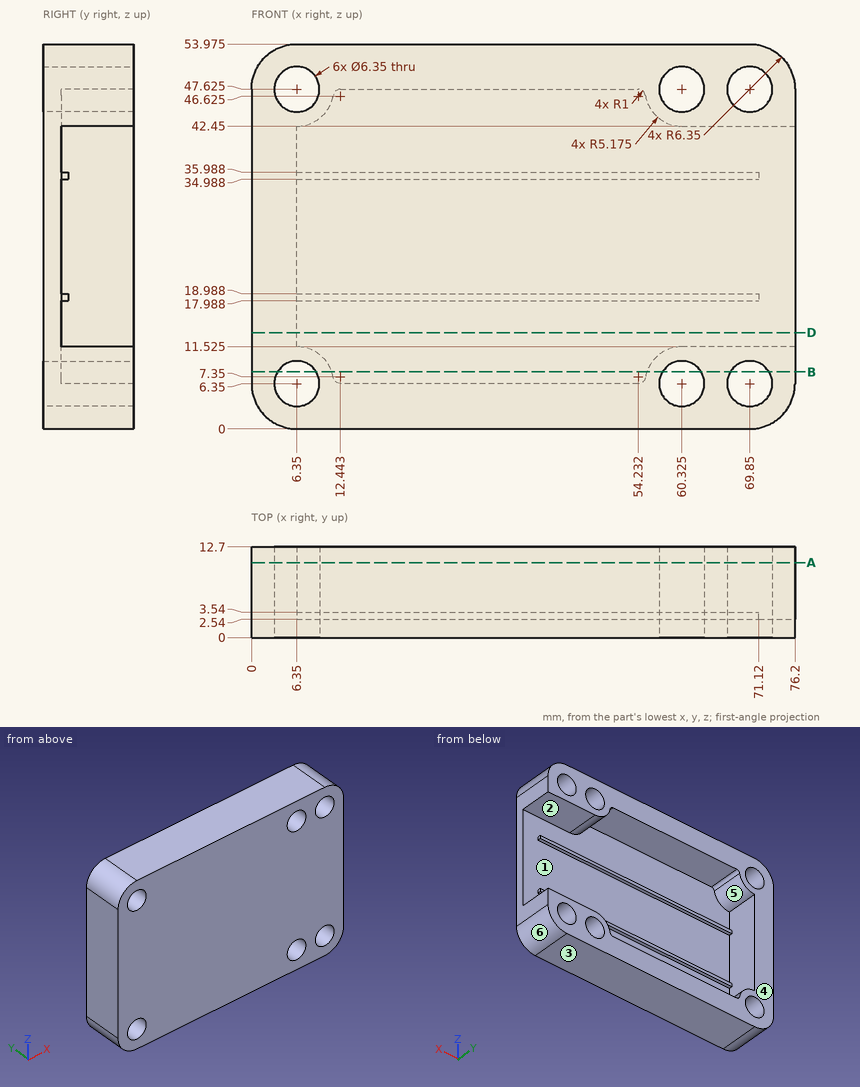
For this review, use the dimensioned drawing (mm, ordinates from the lowest corner) and the shaded views. A direction names the side the tool comes from. Give positions to 0.01 mm unless a question says otherwise; leave off trailing zeros. Loops run counter-clockwise (first coordinate to the right, second up) from the corner with the lowest first, then second, coordinate; pieces in that order, holes last. Notation, with made-up numbers: (58.25, 11) -> (94.25, 11) arc R16 cw to (94.25, 17) -> close; hole circle Ø2 at (31, -18.75). An arc over 180 degrees is marked (long way). One line per question, with ' | ' between items. Start each with the question number.
(1) We need section B-B (z = 8). State the section outline as (x, y) points (1 decimal).
(2) Draft analysis for pull direction X (two halves, no side actions). For the marked faces 4, 5 and 6, state which applies: +X half, -X half, draft (parallel to the pull), parting line (faces both ways), or undercut.
(3) We need section D-D (z = 13.5). State the section outline as (x, y) points.
(4) For line 1 (X direction, y = 9.75, z = 9) (1 decimal); line 2 (X direction, y = 11.25, z = 48); line 3 (X direction, y = 8.5, z = 30), list the stretches that pass through material, from the lowest coordinate up.
(5) We need section A-A (y = 10.5). State how many separate pieces and enclosed holes the cut face has, and give its area (3 significant figures).
(6) Insertion check: P1, Ø4, axis at x = 6.35, z = 47.625, coming from the -Y side; P2, Ø0.5, axis at y = 3, z = 18.5, coming from the +X side; P3, Ø6, axis at x = 17.5, z = 12.5, coming from the +Y side; P4, Ø0.8, axis at x = 32, z = 18.5, coming from the +Y side. Each pin has a flat end and moves straight along its axis. Give the tip position at first contact, or say it passes through.
(7) For the marked faces 1, 2 and 3, list the 3-axis set-ups (+Z, -Z, +X, -X, +Y, -Y) from which the entire face can be reached by the end or side of a thin tool; tool diameter is ignored.
The answers:
1) outline: (0, 0) -> (3.6, 0) -> (3.6, 12.7) -> (0, 12.7) -> close; (9.1, 0) -> (57.6, 0) -> (57.6, 12.7) -> (55.4, 12.7) -> (55.4, 2.5) -> (11.3, 2.5) -> (11.3, 12.7) -> (9.1, 12.7) -> close; (63, 0) -> (67.1, 0) -> (67.1, 12.7) -> (63, 12.7) -> close; (72.6, 0) -> (76.2, 0) -> (76.2, 12.7) -> (72.6, 12.7) -> close
2) face 4: draft | face 5: undercut | face 6: +X half
3) outline: (0, 0) -> (76.2, 0) -> (76.2, 2.54) -> (6.35, 2.54) -> (6.35, 12.7) -> (0, 12.7) -> close
4) line 1: x = 0 to 4.6, 8.1 to 10.8, 55.9 to 58.6, 62.1 to 68.1, 71.6 to 76.2 | line 2: x = 0.01 to 3.2, 9.5 to 57.17, 63.48 to 66.7, 73 to 76.19 | line 3: x = 0 to 6.35
5) separate pieces: 1 | enclosed holes: 6 | area: 1,250 mm^2
6) P1: passes through | P2: stops at x = 71.12 | P3: stops at y = 2.54 | P4: stops at y = 3.54
7) face 1: +Y | face 2: +X, +Y | face 3: -Z, +X, -X, +Y, -Y
